```python
from build123d import *

# Parameters (mm, degrees)
SKETCH2_W           = 100
SKETCH2_H           = 50
BOSS_EXTRUDE1_DEPTH = 3
BOSS_EXTRUDE2_DEPTH = 5


with BuildPart() as part:
    # Sketch2 → Boss-Extrude1 (new body)
    with BuildSketch(Plane(origin=(0, 0, 0), x_dir=(1, 0, 0), z_dir=(0, 1, 0))):
        with Locations((50, 25)):
            Rectangle(SKETCH2_W, SKETCH2_H)
    extrude(amount=BOSS_EXTRUDE1_DEPTH)

    # Sketch3 → Boss-Extrude2 (add)
    with BuildSketch(Plane(origin=(0, 3, 0), x_dir=(1, 0, 0), z_dir=(0, 1, 0))):
        Polygon((3, 37), (3, 47), (13, 47), (13, 44), (6, 44), (6, 37), align=None)
        Polygon((13, 3), (3, 3), (3, 13), (6, 13), (6, 6), (13, 6), align=None)
        Polygon((97, 13), (97, 3), (87, 3), (87, 6), (94, 6), (94, 13), align=None)
        Polygon((87, 47), (97, 47), (97, 37), (94, 37), (94, 44), (87, 44), align=None)
    extrude(amount=BOSS_EXTRUDE2_DEPTH)


solid = part.part
```
Geometry check sheet. Reference: the model listing, model coordinates, mm. A direction names the side the tool comes from. Coordinates: 2 decimals unless noted, no trailing zeros. Order: outer loops, then holes, each group sorted by start corner. A loop starts at its lowest first (then second) coordinate and runs counter-clockwise, first axis right, second up.
Item 1: Section check A-A (y = 6.25). Enter the section's corners in (x, z), plus the area to 3 significant figures.
Item 2: Depth check by flat-ended pin: pin 1 (0.9 mm diameter, centred on x = 4.5, y = 5, fed in from -Z); pin 2 (3 mm diameter, centred on x = 46, z = -39, fed in from +Y); pin 3 (3.5 mm diameter, centred on y = 6.5, z = -46, fed in from +X); pin 4 (4 mm diameter, centred on y = 4.5, z = -8, fed in from -X). Enter the tip coordinate at first touch or a pass-through.
Item 3: Section check B-B (x = 90.5). Enter the section's corners in (y, z), plus the area to 3 significant figures.
Item 4: Section check C-C (z = -10). Enter the section's corners in (x, y).
Item 5: Mould release check, pull along Z, two halves, no side actions. Record for faces 6 (the flat face through (6, 5, -41)), 7 (the flat face through (8, 5, -47)), 8 (the flat face through (8, 5, -3)): released by +Z, released by -Z, zero draft, split by the parting line, or undercut.
Item 6: Section check D-D (z = -15.5). Enter the section's corners in (x, y), plus the area to 3 significant figures.
Item 7: Tool access check on faces 1 (the flat face through (13, 5, -5)), 2 (the flat face through (92, 5, -47)), 3 (the flat face through (92, 5, -3)), 4 (the flat face through (9, 5, -6)), 5 (the flat face through (3, 5, -42)). Record the directions out of +Z, -Z, +X, -X, +Y, -Y that give a thin tool (end or side, any length) a straight path to the whole face; none if there is none.
Item 8: Scan lines: line 1 along Z through (x, y) = (89, 4.5); line 2 along Y through (x, z) = (95, -22.5). Record each from-to range of solid material in increasing order.
Check sheet entries:
1. outline: (3, -47) - (13, -47) - (13, -44) - (6, -44) - (6, -37) - (3, -37) - close; (3, -13) - (6, -13) - (6, -6) - (13, -6) - (13, -3) - (3, -3) - close; (87, -47) - (97, -47) - (97, -37) - (94, -37) - (94, -44) - (87, -44) - close; (87, -6) - (94, -6) - (94, -13) - (97, -13) - (97, -3) - (87, -3) - close
1. area: 204 mm2
2. pin 1: stops at z = -47
2. pin 2: stops at y = 3
2. pin 3: stops at x = 97
2. pin 4: stops at x = 0
3. outline: (0, -50) - (3, -50) - (3, -47) - (8, -47) - (8, -44) - (3, -44) - (3, -6) - (8, -6) - (8, -3) - (3, -3) - (3, 0) - (0, 0) - close
3. area: 180 mm2
4. outline: (0, 0) - (100, 0) - (100, 3) - (97, 3) - (97, 8) - (94, 8) - (94, 3) - (6, 3) - (6, 8) - (3, 8) - (3, 3) - (0, 3) - close
5. face 6: undercut
5. face 7: released by -Z
5. face 8: released by +Z
6. outline: (0, 0) - (100, 0) - (100, 3) - (0, 3) - close
6. area: 300 mm2
7. face 1: +Z, -Z, +Y
7. face 2: -Z, +X, -X, +Y
7. face 3: +Z, +X, -X, +Y
7. face 4: +Y
7. face 5: +Z, -Z, -X, +Y
8. line 1: z = -47 to -44, -6 to -3
8. line 2: y = 0 to 3
